```python
from build123d import *

# Parameters (mm, degrees)
SKETCH3_R               = 11.7
CUT_EXTRUDE1_DEPTH      = 1
CUT_EXTRUDE1_DEPTH_BACK = 301


with BuildPart() as part:
    # Sketch1 → Revolve1 (revolve)
    with BuildSketch(Plane.XY):
        Polygon((-150, 0), (150, 0), (150, 12.7), (75, 12.7), (75, 13.7), (72, 13.7), (72, 12.7), (-72, 12.7), (-72, 13.7), (-75, 13.7), (-75, 12.7), (-150, 12.7), align=None)
    revolve(axis=Axis((-150, 0, 0), (1, 0, 0)))

    # Sketch3 → Cut-Extrude1 (cut, two sides)
    with BuildSketch(Plane(origin=(150, 0, 0), x_dir=(0, 0, -1), z_dir=(1, 0, 0))) as cut_extrude1_sk:
        Circle(SKETCH3_R)
    extrude(amount=CUT_EXTRUDE1_DEPTH, mode=Mode.SUBTRACT)
    extrude(cut_extrude1_sk.sketch, amount=-CUT_EXTRUDE1_DEPTH_BACK, mode=Mode.SUBTRACT)


solid = part.part
```
Read the model definition and answer for the solid it produces. Units are mm, in the model's axes. A direction names the side the tool comes from. Give positions to 0.01 mm unless a question says otherwise; leave off trailing zeros. Write each loop counter-clockwise with the first axis right and the second up, starting at its lowest first coordinate (ties: lowest second). Pieces come first, ordered by that corner, then holes. Notation, with made-up numbers: (36.5, 25) -> (83.5, 25) arc R7 ccw to (83.5, 36) -> close; hole circle Ø6 at (26.5, 79.25). An arc over 180 degrees is marked (long way). Answer in a Markdown table with one row per item.
1) Determine the mould class of faces 1 (the cylindrical face through (73.479, -10.097, 9.259)), 2 (the cylindrical face through (2.1, -11.42, 2.54)), 3 (the flat face through (-150, 8.4, -8.4)) for opening direction Y: released by +Y, released by -Y, zero draft, split by the parting line, or undercut.
Results list:
| item | result |
|---|---|
| face 1 | split by the parting line |
| face 2 | undercut |
| face 3 | zero draft |
2) Straight lines are drawn through the part: line 1 (Y direction, x = -67, z = 0.5); line 2 (X direction, y = 12.5, z = 4.25); line 3 (Y direction, x = -68, z = -6.25). For each, find the intervals that lie inside material, in ascending order. Write a range as [from, to].
Results list:
| item | result |
|---|---|
| line 1 | [-12.69, -11.69], [11.69, 12.69] |
| line 2 | [-75, -72], [72, 75] |
| line 3 | [-11.06, -9.89], [9.89, 11.06] |
3) A tool of negligible diameter and unlimited length cuts with its end or side. For faces 4 (the flat face through (-75, 9.1, -9.1)), 5 (the flat face through (-72, -9.1, -9.1)), 6 (the cylindrical face through (111.98, -2.75, -12.4)), 7 (the flat face through (150, -8.4, -8.4)), 8 (the cylindrical face through (-73.521, -10.097, 9.259)), from which of +Z, -Z, +X, -X, +Y, -Y can it reach the whole face along a straight path? Write none if from no direction.
Results list:
| item | result |
|---|---|
| face 4 | -X |
| face 5 | none |
| face 6 | +X |
| face 7 | +Z, -Z, +X, +Y, -Y |
| face 8 | +X, -X |
4) Section A-A on y = 0 is taken. Give the vertices of the cut face in (x, z).
Results list:
| item | result |
|---|---|
| outline | (-150, -12.7) -> (-75, -12.7) -> (-75, -13.7) -> (-72, -13.7) -> (-72, -12.7) -> (72, -12.7) -> (72, -13.7) -> (75, -13.7) -> (75, -12.7) -> (150, -12.7) -> (150, -11.7) -> (-150, -11.7) -> close; (-150, 11.7) -> (150, 11.7) -> (150, 12.7) -> (75, 12.7) -> (75, 13.7) -> (72, 13.7) -> (72, 12.7) -> (-72, 12.7) -> (-72, 13.7) -> (-75, 13.7) -> (-75, 12.7) -> (-150, 12.7) -> close |
5) Section C-C on x = -37.5 is taken. Give the vertices of the cut face in (y, z), plus the area to 3 significant figures.
Results list:
| item | result |
|---|---|
| outline | circle Ø25.4 at (0, 0); hole circle Ø23.4 at (0, 0) |
| area | 76.7 mm^2 |
6) Each of these flat-tipped pins is pushed along its axis until it touches: pin 1 Ø12 at (y, z) = (-5.5, -1) entering from -X; pin 2 Ø1.5 at (x, z) = (-75, -6) entering from +Y; pin 3 Ø8 at (x, y) = (-26.5, -9) entering from +Z; pin 4 Ø4 at (x, z) = (-7.5, -1.5) entering from -Y. Where does it stop, or does it pass through?
Results list:
| item | result |
|---|---|
| pin 1 | through |
| pin 2 | y = 12.65 |
| pin 3 | z = 11.67 |
| pin 4 | y = -12.7 |
